Here's how the part is built. I have some questions about the finished solid (model axes, mm). Round coordinates to 2 decimals unless told otherwise and drop trailing zeros. Use a Markdown table: item, result.
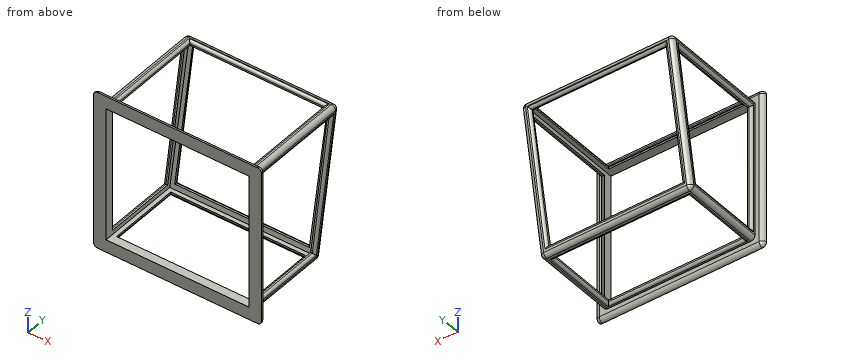
```python
from build123d import *

# Parameters (mm, degrees)
SKETCH1_W           = 180
SKETCH1_H           = 168.6
SKETCH1_W_2         = 170
SKETCH1_H_2         = 158.6
BOSS_EXTRUDE1_DEPTH = 135
SKETCH1_3_W         = 170
SKETCH1_3_H         = 158.6
SKETCH1_3_W_2       = 160
SKETCH1_3_H_2       = 148.6
BOSS_EXTRUDE2_DEPTH = 135
CUT_EXTRUDE1_DEPTH  = 180
SKETCH3_W           = 160
SKETCH3_H           = 151.248240867
CUT_EXTRUDE2_DEPTH  = 10
SKETCH4_W           = 170
SKETCH4_H           = 158.6
CUT_EXTRUDE3_DEPTH  = 100
CUT_EXTRUDE5_DEPTH  = 170
CUT_EXTRUDE6_DEPTH  = 180
SKETCH7_W           = 160
SKETCH7_H           = 115
CUT_EXTRUDE7_DEPTH  = 10
SKETCH8_W           = 160
SKETCH8_H           = 85
CUT_EXTRUDE8_DEPTH  = 10
FILLET2_R           = 3
FILLET3_R           = 3
SKETCH9_W           = 180
SKETCH9_H           = 5
BOSS_EXTRUDE3_DEPTH = 10
SKETCH10_W          = 180
SKETCH10_H          = 5
BOSS_EXTRUDE4_DEPTH = 10
SKETCH11_W          = 188.6
SKETCH11_H          = 5
BOSS_EXTRUDE5_DEPTH = 10
SKETCH12_W          = 188.6
SKETCH12_H          = 5
BOSS_EXTRUDE6_DEPTH = 10
FILLET4_R           = 5
FILLET5_R           = 5


with BuildPart() as part:
    # Sketch1 → Boss-Extrude1 (new body)
    with BuildSketch(Plane(origin=(0, 0, 0), x_dir=(1, 0, 0), z_dir=(0, 1, 0))):
        with Locations((85, 79.3)):
            Rectangle(SKETCH1_W, SKETCH1_H)
        with Locations((85, 79.3)):
            Rectangle(SKETCH1_W_2, SKETCH1_H_2, mode=Mode.SUBTRACT)
    extrude(amount=BOSS_EXTRUDE1_DEPTH)

    # Sketch1<3> → Boss-Extrude2 (add)
    # profile 1 of 2: a face of its own
    with BuildSketch(Plane(origin=(0, 0, 0), x_dir=(1, 0, 0), z_dir=(0, 1, 0))):
        with Locations((85, 79.3)):
            Rectangle(SKETCH1_3_W, SKETCH1_3_H)
        with Locations((85, 79.3)):
            Rectangle(SKETCH1_3_W_2, SKETCH1_3_H_2, mode=Mode.SUBTRACT)
    # profile 2 of 2: a face of its own
    with BuildSketch(Plane(origin=(0, 0, 0), x_dir=(1, 0, 0), z_dir=(0, 1, 0))):
        with Locations((85, 79.3)):
            Rectangle(SKETCH1_3_W_2, SKETCH1_3_H_2)
    extrude(amount=BOSS_EXTRUDE2_DEPTH)

    # Sketch2 → Cut-Extrude1 (cut)
    with BuildSketch(Plane(origin=(175, 0, 0), x_dir=(0, 0, -1), z_dir=(1, 0, 0))):
        Polygon((-5, 135), (163.6, 135), (163.6, 105), align=None)
    extrude(amount=-CUT_EXTRUDE1_DEPTH, mode=Mode.SUBTRACT)

    # Sketch3 → Cut-Extrude2 (cut)
    with BuildSketch(Plane(origin=(0, 129.994537263, -23.130700581), x_dir=(1, 0, 0), z_dir=(0, 0.9845356609009732, -0.17518428129910554))):
        with Locations((85, 57.051564154)):
            Rectangle(SKETCH3_W, SKETCH3_H)
    extrude(amount=-CUT_EXTRUDE2_DEPTH, mode=Mode.SUBTRACT)

    # Sketch4 → Cut-Extrude3 (cut)
    with BuildSketch(Plane.XZ):
        with Locations((85, -79.3)):
            Rectangle(SKETCH4_W, SKETCH4_H)
    extrude(amount=-CUT_EXTRUDE3_DEPTH, mode=Mode.SUBTRACT)

    # Sketch5 → Cut-Extrude5 (cut)
    with BuildSketch(Plane(origin=(0, 0, 0), x_dir=(0, 0, -1), z_dir=(1, 0, 0))):
        Polygon((0, 130), (158.6, 100), (0, 100), align=None)
    extrude(amount=CUT_EXTRUDE5_DEPTH, mode=Mode.SUBTRACT)

    # Sketch6 → Cut-Extrude6 (cut)
    with BuildSketch(Plane(origin=(175, 0, 0), x_dir=(0, 0, -1), z_dir=(1, 0, 0))):
        Polygon((5, 10), (153.6, 10), (153.6, 96.622287019), (5, 123.063568157), align=None)
    extrude(amount=-CUT_EXTRUDE6_DEPTH, mode=Mode.SUBTRACT)

    # Sketch7 → Cut-Extrude7 (cut)
    with BuildSketch(Plane.XY.offset(5)):
        with Locations((85, 67.5)):
            Rectangle(SKETCH7_W, SKETCH7_H)
    extrude(amount=-CUT_EXTRUDE7_DEPTH, mode=Mode.SUBTRACT)

    # Sketch8 → Cut-Extrude8 (cut)
    with BuildSketch(Plane(origin=(0, 0, -163.6), x_dir=(-1, 0, 0), z_dir=(0, 0, -1))):
        with Locations((-85, 52.5)):
            Rectangle(SKETCH8_W, SKETCH8_H)
    extrude(amount=-CUT_EXTRUDE8_DEPTH, mode=Mode.SUBTRACT)

    # Fillet2
    fillet2_edges = [part.edges().sort_by_distance(p)[0] for p in [
        (85, 106.751842813, -153.754643391),
        (165, 120, -79.3),
        (5, 120, -79.3),
        (85, 133.248157187, -4.845356609),
    ]]
    fillet(fillet2_edges, radius=FILLET2_R)

    # Fillet3
    fillet3_edges = [part.edges().sort_by_distance(p)[0] for p in [
        (-5, 10, -79.3),
        (-5, 66.531784079, -5),
        (-5, 109.842927588, -79.3),
        (-5, 53.311143509, -153.6),
        (175, 10, -79.3),
        (175, 53.311143509, -153.6),
        (175, 109.842927588, -79.3),
        (175, 66.531784079, -5),
        (165, 67.5, 5),
        (85, 10, 5),
        (85, 125, 5),
        (5, 67.5, 5),
        (85, 95, -163.6),
        (5, 52.5, -163.6),
        (165, 52.5, -163.6),
        (85, 10, -163.6),
    ]]
    fillet(fillet3_edges, radius=FILLET3_R)

    # Sketch9 → Boss-Extrude3 (add)
    with BuildSketch(Plane(origin=(0, 0, -163.6), x_dir=(-1, 0, 0), z_dir=(0, 0, -1))):
        with Locations((-85, 2.5)):
            Rectangle(SKETCH9_W, SKETCH9_H)
    extrude(amount=BOSS_EXTRUDE3_DEPTH)

    # Sketch10 → Boss-Extrude4 (add)
    with BuildSketch(Plane.XY.offset(5)):
        with Locations((85, 2.5)):
            Rectangle(SKETCH10_W, SKETCH10_H)
    extrude(amount=BOSS_EXTRUDE4_DEPTH)

    # Sketch11 → Boss-Extrude5 (add)
    with BuildSketch(Plane.ZY.offset(5)):
        with Locations((-79.3, 2.5)):
            Rectangle(SKETCH11_W, SKETCH11_H)
    extrude(amount=BOSS_EXTRUDE5_DEPTH)

    # Sketch12 → Boss-Extrude6 (add)
    with BuildSketch(Plane(origin=(175, 0, 0), x_dir=(0, 0, -1), z_dir=(1, 0, 0))):
        with Locations((79.3, 2.5)):
            Rectangle(SKETCH12_W, SKETCH12_H)
    extrude(amount=BOSS_EXTRUDE6_DEPTH)

    # Fillet4
    fillet4_edges = [part.edges().sort_by_distance(p)[0] for p in [
        (85, 135, 5),
        (175, 70, 5),
        (-5, 70, 5),
        (-5, 55, -163.6),
        (175, 55, -163.6),
        (-5, 120, -79.3),
        (85, 105, -163.6),
        (175, 120, -79.3),
    ]]
    fillet(fillet4_edges, radius=FILLET4_R)

    # Fillet5
    fillet5_edges = [part.edges().sort_by_distance(p)[0] for p in [
        (85, 5, -173.6),
        (85, 5, 15),
        (-15, 2.5, -173.6),
        (-15, 2.5, 15),
        (-15, 5, -79.3),
        (185, 2.5, 15),
        (185, 2.5, -173.6),
        (185, 5, -79.3),
    ]]
    fillet(fillet5_edges, radius=FILLET5_R - 0.0001)  # a hair under: the kernel refuses the full size


solid = part.part
```
Q1. Will these pins go through, and if not, where does the flat tip stop? P1, Ø2, axis at x = 170.5, y = 44, coming from the -Z side; P2, Ø1.6, axis at y = 84, z = 1.5, coming from the -X side; P3, Ø2, axis at x = -1, z = -103.5, coming from the +Y side.
Return value:
| item | result |
|---|---|
| P1 | stops at z = -163.6 |
| P2 | stops at x = -4.95 |
| P3 | stops at y = 115.82 |
Q2. I need wall thicknesses on line 1 (Z direction, x = 168.5, y = 33.5); line 2 (Y direction, x = 176.5, z = -33); line 3 (Y direction, x = 171.5, z = -136). Which ranges of each line are inside material? Lowest first, please. Write a range as from..to.
Return value:
| item | result |
|---|---|
| line 1 | z = -163.6..-158.6, 0..5 |
| line 2 | y = 0..5 |
| line 3 | y = 0..10, 99.75..109.68 |
Q3. Imagine slicing it at A-A, the plane y = 24.5. Give the number of separate pieces and of enclosed holes in the cut face, then the cut area to 3 significant figures.
Return value:
| item | result |
|---|---|
| separate pieces | 4 |
| enclosed holes | 0 |
| area | 263 mm^2 |
